Work out the finished part from the listing and answer in its coordinate system (mm). Face numbers are marked on the shaded views. A direction names the side the tool comes from. Round coordinates to 2 decimals unless told otherwise and drop trailing zeros.
from build123d import *

# Parameters (mm, degrees)
BOSS_EXTRUDE1_DEPTH = 12


with BuildPart() as part:
    # Sketch1 → Boss-Extrude1 (new body)
    with BuildSketch(Plane.XY):
        Polygon((1.001450614, 7.5), (0.749315442, 8.669732015), (0.301638962, 9.779430578), (-0.301638962, 9.779430578), (-0.749315442, 8.669732015), (-1.001450614, 7.5), (-1.998549386, 7.5), (-2.250684558, 8.669732015), (-2.698361038, 9.779430578), (-3.301638962, 9.779430578), (-3.749315442, 8.669732015), (-4.001450614, 7.5), (-4.998549386, 7.5), (-5.250684558, 8.669732015), (-5.698361038, 9.779430578), (-6.301638962, 9.779430578), (-6.749315442, 8.669732015), (-7.001450614, 7.5), (-7.998549386, 7.5), (-8.250684558, 8.669732015), (-8.698361038, 9.779430578), (-9.301638962, 9.779430578), (-9.749315442, 8.669732015), (-10.001450614, 7.5), (-10.998549386, 7.5), (-11.250684558, 8.669732015), (-11.698361038, 9.779430578), (-12.301638962, 9.779430578), (-12.749315442, 8.669732015), (-13.001450614, 7.5), (-13.998549386, 7.5), (-14.250684558, 8.669732015), (-14.698361038, 9.779430578), (-15.301638962, 9.779430578), (-15.749315442, 8.669732015), (-16.001450614, 7.5), (-16.998549386, 7.5), (-17.250684558, 8.669732015), (-17.698361038, 9.779430578), (-18.301638962, 9.779430578), (-18.749315442, 8.669732015), (-19.001450614, 7.5), (-19.998549386, 7.5), (-20.250684558, 8.669732015), (-20.698361038, 9.779430578), (-21.301638962, 9.779430578), (-21.749315442, 8.669732015), (-22.001450614, 7.5), (-22.998549386, 7.5), (-23.250684558, 8.669732015), (-23.698361038, 9.779430578), (-24.301638962, 9.779430578), (-24.749315442, 8.669732015), (-25.001450614, 7.5), (-25.998549386, 7.5), (-26.250684558, 8.669732015), (-26.698361038, 9.779430578), (-27.301638962, 9.779430578), (-27.749315442, 8.669732015), (-28.001450614, 7.5), (-28.998549386, 7.5), (-29.250684558, 8.669732015), (-29.698361038, 9.779430578), (-30.301638962, 9.779430578), (-30.749315442, 8.669732015), (-31.001450614, 7.5), (-50, 7.5), (-50, -7.5), (50, -7.5), (50, 7.5), (34.001450614, 7.5), (33.749315442, 8.669732015), (33.301638962, 9.779430578), (32.698361038, 9.779430578), (32.250684558, 8.669732015), (31.998549386, 7.5), (31.001450614, 7.5), (30.749315442, 8.669732015), (30.301638962, 9.779430578), (29.698361038, 9.779430578), (29.250684558, 8.669732015), (28.998549386, 7.5), (28.001450614, 7.5), (27.749315442, 8.669732015), (27.301638962, 9.779430578), (26.698361038, 9.779430578), (26.250684558, 8.669732015), (25.998549386, 7.5), (25.001450614, 7.5), (24.749315442, 8.669732015), (24.301638962, 9.779430578), (23.698361038, 9.779430578), (23.250684558, 8.669732015), (22.998549386, 7.5), (22.001450614, 7.5), (21.749315442, 8.669732015), (21.301638962, 9.779430578), (20.698361038, 9.779430578), (20.250684558, 8.669732015), (19.998549386, 7.5), (19.001450614, 7.5), (18.749315442, 8.669732015), (18.301638962, 9.779430578), (17.698361038, 9.779430578), (17.250684558, 8.669732015), (16.998549386, 7.5), (16.001450614, 7.5), (15.749315442, 8.669732015), (15.301638962, 9.779430578), (14.698361038, 9.779430578), (14.250684558, 8.669732015), (13.998549386, 7.5), (13.001450614, 7.5), (12.749315442, 8.669732015), (12.301638962, 9.779430578), (11.698361038, 9.779430578), (11.250684558, 8.669732015), (10.998549386, 7.5), (10.001450614, 7.5), (9.749315442, 8.669732015), (9.301638962, 9.779430578), (8.698361038, 9.779430578), (8.250684558, 8.669732015), (7.998549386, 7.5), (7.001450614, 7.5), (6.749315442, 8.669732015), (6.301638962, 9.779430578), (5.698361038, 9.779430578), (5.250684558, 8.669732015), (4.998549386, 7.5), (4.001450614, 7.5), (3.749315442, 8.669732015), (3.301638962, 9.779430578), (2.698361038, 9.779430578), (2.250684558, 8.669732015), (1.998549386, 7.5), align=None)
    extrude(amount=BOSS_EXTRUDE1_DEPTH)


solid = part.part
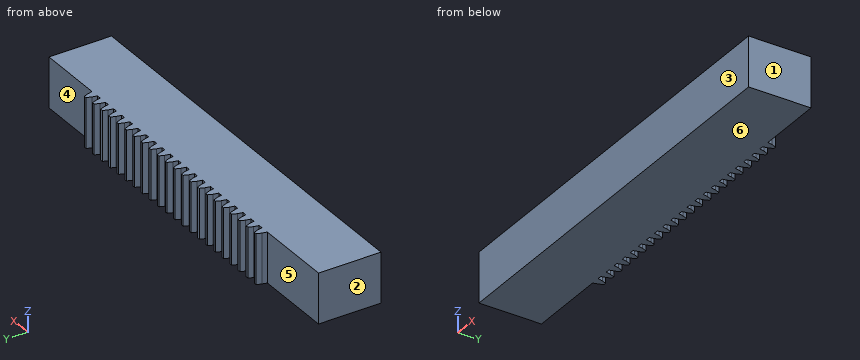
Item 1: For the marked faces 4, 5 and 6, determine the directions among +Z, -Z, +X, -X, +Y, -Y from which every point of the face is accessible in a straight line to the end or side of a thin tool.
Item 2: This flat-tipped pin is pushed along its axis until it touches: P1, Ø0.8, axis at x = -7.5, z = 6.5, coming from the +Y side. Where does it stop, or does it pass through?
Item 3: Determine the mould class of the marked faces 1, 2 and 3 for opening direction X: pulls with the +X half, pulls with the -X half, needs draft (parallel to the pull), parting line crosses it, or undercut.
Item 4: Straight lines are drawn through the part: line 1 (Y direction, x = -36, z = 2.75); line 2 (Y direction, x = 12.5, z = 9.75). For each, find the intervals that lie inside material, in ascending order.
Answer below:
1. face 4: +Z, -Z, +X, +Y
1. face 5: +Z, -Z, -X, +Y
1. face 6: -Z, +X, -X, +Y, -Y
2. P1: stops at y = 7.5
3. face 1: pulls with the +X half
3. face 2: pulls with the -X half
3. face 3: needs draft
4. line 1: y = -7.5 to 7.5
4. line 2: y = -7.5 to 9.29
